The drawing under review shows one solid part. Ordinate dimensions are in mm from its lowest x, y, z. A direction names the side the tool comes from. Round coordinates to 2 decimals unless told otherwise and drop trailing zeros. Write each loop counter-clockwise with the first axis right and the second up, starting at its lowest first coordinate (ties: lowest second). Pieces come first, ordered by that corner, then holes. Notation, with made-up numbers: M 42.25,73 L 67.25,73 A13 ccw 67.25,92 Z; hole C 7.25,2.5 d4. An arc over 180 degrees is marked long. Write item = value, one per line. Start each with the question number.
Item 1: Take a section at C-C, the plane z = 3.25. Give the boundary of the cut face in (x, y), plus the area to 3 significant figures.
Item 2: Tool access review of the marked faces 4 and 5: name each direction out of +Z, -Z, +X, -X, +Y, -Y from which nothing blocks a thin tool from reaching the whole face with its end or side.
Item 3: Take a section at A-A, the plane x = 8. Give the boundary of the cut face in (y, z).
Item 4: For pin 1 Ø3 at (x, z) = (3.5, 3) entering from -Y; pin 2 Ø1.5 at (y, z) = (5.5, 2) entering from +X; pin 3 Ø4 at (x, y) = (8, 8) entering from +Z; pin 4 Ø1 at (x, z) = (12, 4.5) entering from -Y, all flat-tipped, find the tip position at first contact; note any pin that passes through.
Item 5: Take a section at D-D, the plane y = 2.5. Give the boundary of the cut face in (x, z), plus the area to 3 significant figures.
Item 6: To check wall thickness, follow line 1 along Z through (x, y) = (13.75, 13.5); line 2 along Y through (x, z) = (8, 11.75); line 3 along Y through (x, z) = (8, 7.5). State the ranges of each line that lie inside material, in increasing order.
Item 7: The part is to be moulded in two halves that separate along Z. For the marked faces 1, 2 and 3, say which applies: +Z half, -Z half, draft (parallel to the pull), parting line (faces both ways), or undercut.
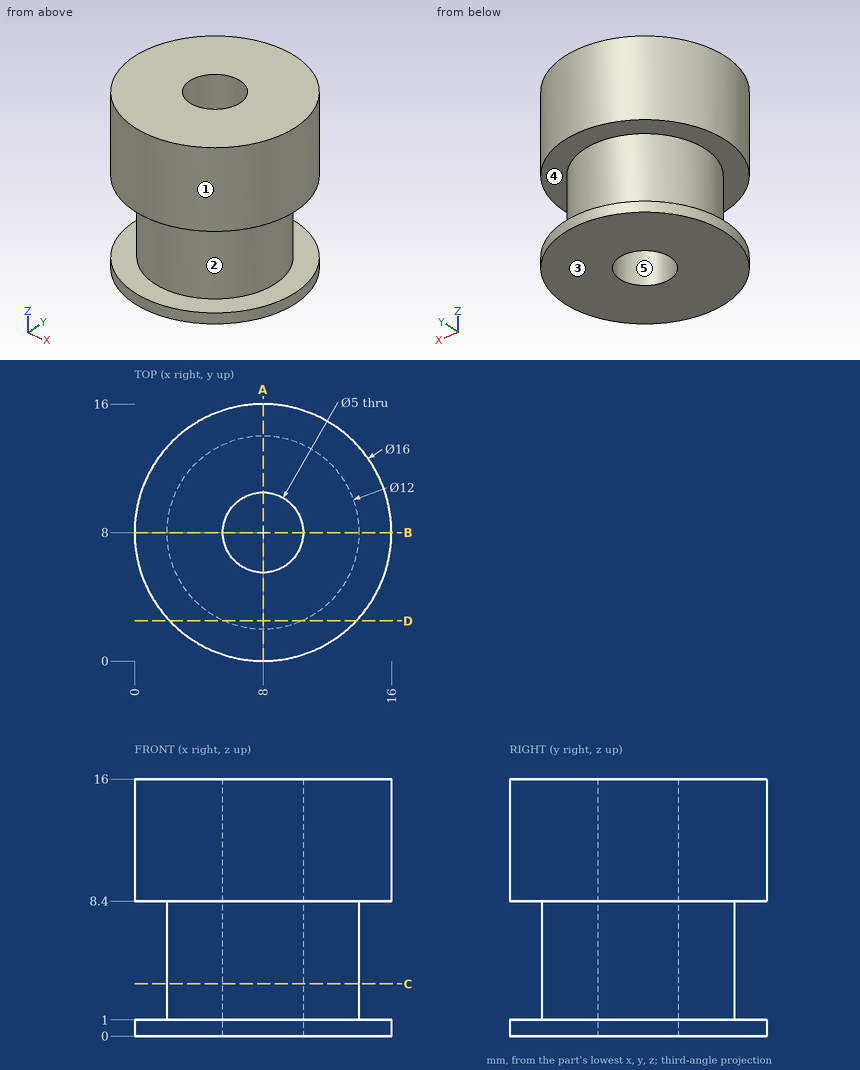
Response values:
q1.outline = C 8,8 d12; hole C 8,8 d5
q1.area = 93.5 mm2
q2.face_4 = none
q2.face_5 = +Z, -Z
q3.outline = M 0,0 L 5.5,0 L 5.5,16 L 0,16 L 0,8.4 L 2,8.4 L 2,1 L 0,1 Z; M 10.5,0 L 16,0 L 16,1 L 14,1 L 14,8.4 L 16,8.4 L 16,16 L 10.5,16 Z
q4.pin_1 = 2.8
q4.pin_2 = 13.74
q4.pin_3 = through
q4.pin_4 = 3.13
q5.outline = M 2.19,0 L 13.81,0 L 13.81,1 L 10.4,1 L 10.4,8.4 L 13.81,8.4 L 13.81,16 L 2.19,16 L 2.19,8.4 L 5.6,8.4 L 5.6,1 L 2.19,1 Z
q5.area = 135 mm2
q6.line_1 = 0 to 1, 8.4 to 16
q6.line_2 = 0 to 5.5, 10.5 to 16
q6.line_3 = 2 to 5.5, 10.5 to 14
q7.face_1 = draft
q7.face_2 = undercut
q7.face_3 = -Z half
